Check sheet for the modelled part. Datum: model origin and axes. Units: mm. A direction names the side the tool comes from. Round coordinates to 2 decimals unless told otherwise and drop trailing zeros. Write each loop counter-clockwise with the first axis right and the second up, starting at its lowest first coordinate (ties: lowest second). Pieces come first, ordered by that corner, then holes.
Item 1: Release check for a two-part mould opening along Y. For faces 1 (the cylindrical face through (-20.789, -12.087, 3.413)), 2 (the cylindrical face through (-0.073, 24.047, 3.413)), 3 (the cylindrical face through (-9.556, 5.276, 3.318)) record: +Y half, -Y half, draft (parallel to the pull), parting line (faces both ways), or undercut.
Item 2: Material ranges on line 1 (X direction, y = -28.5, z = 6.25); line 2 (X direction, y = -27.5, z = 1); line 3 (Z direction, x = 0, y = 4), recorded low to high.
Item 3: Cross-section at D-D on y = -4. Enter the section's corners in (x, z).
Item 4: Tool access check on faces 4 (the cylindrical face through (-10.1, -33.28, 3.32)), 5 (the flat face through (19.486, -23, 3)), 6 (the flat face through (-2, -2, 3.6)). Record the directions out of +Z, -Z, +X, -X, +Y, -Y that give a thin tool (end or side, any length) a straight path to the whole face; none if there is none.
Item 5: Cross-section at C-C on z = 4.75. Count the separate pieces of the cut face and the enclosed holes in it, plus the area to 3 significant figures.
Item 6: Go/stop test with flat-tipped pins: pin 1 Ø2.5 at (x, y) = (0, -12.5) entering from -Z; pin 2 Ø1.5 at (y, z) = (4.5, 3.5) entering from -X; pin 3 Ø5 at (x, y) = (-1.5, 1.5) entering from -Z; pin 4 Ø1 at (x, z) = (-29, 1) entering from +Y. Record where each tip stops, or that it passes through.
Item 7: Cross-section at A-A on x = 6. Enter the section's corners in (y, z).
Item 8: Cross-section at B-B on y = 22.5. Enter the section's corners in (x, z), plus the area to 3 significant figures.
Autodesk Inventor part; units mm, degrees
ref_plane "YZ Plane" through (0, 0, 0) normal (1, 0, 0) x (0, 1, 0)
ref_plane "XZ Plane" through (0, 0, 0) normal (0, 1, 0) x (-1, 0, 0)
ref_plane "XY Plane" through (0, 0, 0) normal (0, 0, 1) x (1, 0, 0)
sketch "Sketch1" plane through (0, 0, 0) normal (0, 0, 1) x (1, 0, 0)
  line L0 (0, 0) -> (-33.403, 19.2853)
  line L1 (0, 0) -> (33.403, 19.2853)
  arc A0 (1.8187, 1.05) -> (-1.8187, 1.05) centre (0, 0) ccw
  circle A1 centre (-20, 22.5) radius 4.75
  circle A2 centre (20, 22.5) radius 4.75
  line L2 (0, 0) -> (-27.7881, 0)
  line L3 (-33.403, 19.2853) -> (-23.6603, 36.1603)
  line L4 (23.6603, 36.1603) -> (33.403, 19.2853)
  line L5 (-23.6603, 36.1603) -> (0, 22.5)
  line L6 (0, 22.5) -> (23.6603, 36.1603)
  dimension "d0" = 120
  dimension "d1" = 2.1
  dimension "d2" = 9.5
  dimension "d3" = 40
  dimension "d4" = 20
  dimension "d5" = 22.5
  dimension "d6" = 30
  dimension "d10" = 10
  dimension "d30" = 10
extrude "Extrusion1" add sketch "Sketch1" along normal blind 6.731 contours L0 L3 L5 L6 L4 L1 A0
fillet "Fillet1" radius 10 3 edges at (-23.6603, 36.1603, 3.3655) (23.6603, 36.1603, 3.3655) (0, 22.5, 3.3655)
pattern_circular "Circular Pattern1" count 3 over 360 about axis through (0, 0, 0) along (0, 0, 1) of "Extrusion1", "Fillet1"
sketch "Sketch2" plane through (0, 0, 0) normal (0, 0, -1) x (-1, 0, 0)
  circle A0 centre (0, 0) radius 2.1
  circle A1 centre (10.8253, 6.25) radius 1.6
  line L0 (19.4856, -17.0235) -> (19.4856, -28.5705)
  line L1 (10.8253, 6.25) -> (0, 0) construction
  line L2 (0, 0) -> (15.25, 0) construction
  point P0 (19.4856, -18.9295)
  dimension "d18" = 3.2
  dimension "d20" = 12.5
  dimension "d33" = 30
extrude "Extrusion2" cut sketch "Sketch2" against normal up to next contours A1
pattern_circular "Circular Pattern2" count 3 over 360 about axis through (0, 0, 0) along (0, 0, 1) of "Extrusion2"
sketch "Sketch3" plane through (0, 0, 0) normal (0, 0, -1) x (-1, 0, 0)
  circle A0 centre (0, 0) radius 2.1
  circle A1 centre (0, 0) radius 8
  dimension "d26" = 16
extrude "Extrusion3" cut sketch "Sketch3" against normal blind 3.6
equation "\"d2\" = MAGDIA"
equation "\"d4\" = 0.5 * d3"
equation "\"d30\" = d10"
equation "\"d12\" = THICKB"
equation "\"d21\" = THICKB"
equation "\"THICKA\" = 3.175"
equation "\"THICKB\" = 6.731"
equation "\"THICKC\" = 12.7"
equation "\"MAGDIA\" = 9.5"
equation "\"BALLDIA\" = 12"
equation "\"THICKPLY\" = 5"
properties part number "Effector_Platform_V2"
Response values:
1. face 1: -Y half
1. face 2: +Y half
1. face 3: undercut
2. line 1: x = -19.49 to -14.24, -4.74 to 4.74, 14.24 to 19.49
2. line 2: x = -19.49 to -14.11, -4.86 to 4.86, 14.11 to 19.49
2. line 3: z = 3.6 to 6.73
3. outline: (-32.04, 0) - (-6.93, 0) - (-6.93, 3.6) - (6.93, 3.6) - (6.93, 0) - (32.04, 0) - (32.04, 6.73) - (-32.04, 6.73) - close
4. face 4: +Z, -Z
4. face 5: +Z, -Z, +X, -Y
4. face 6: -Z
5. separate pieces: 1
5. enclosed holes: 10
5. area: 3,280 mm2
6. pin 1: passes through
6. pin 2: stops at x = -39.45
6. pin 3: stops at z = 3.6
6. pin 4: stops at y = 27.77
7. outline: (-38.57, 0) - (-31.8, 0) - (-31.8, 6.73) - (-38.57, 6.73) - close; (-25.34, 0) - (-5.29, 0) - (-5.29, 3.6) - (5.29, 3.6) - (5.29, 0) - (25.96, 0) - (25.96, 6.73) - (-25.34, 6.73) - close
8. outline: (-31.55, 0) - (-24.75, 0) - (-24.75, 6.73) - (-31.55, 6.73) - close; (-15.25, 0) - (15.25, 0) - (15.25, 6.73) - (-15.25, 6.73) - close; (24.75, 0) - (31.55, 0) - (31.55, 6.73) - (24.75, 6.73) - close
8. area: 297 mm2
